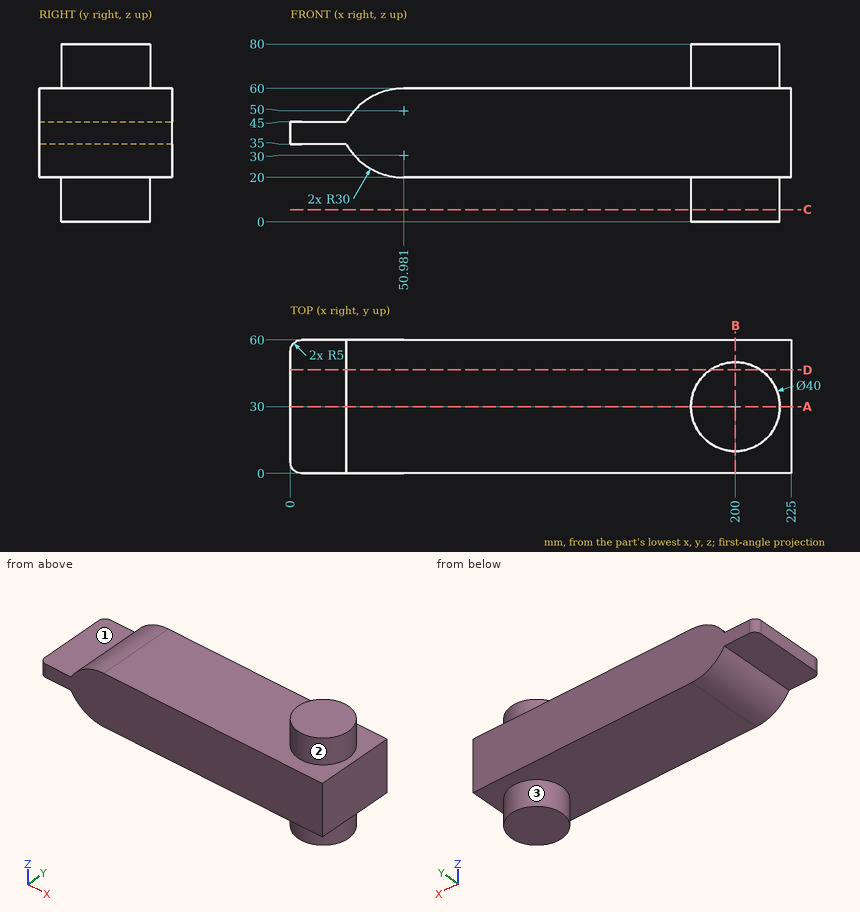
Source: three-view drawing plus pictorial views. Frame: mm from the lowest corner of the part. A direction names the side the tool comes from. Round coordinates to 2 decimals unless told otherwise and drop trailing zeros. Order: outer loops, then holes, each group sorted by start corner. A loop starts at its lowest first (then second) coordinate and runs counter-clockwise, first axis right, second up. Notation, with made-up numbers: (-38.75, -33) - (-21.75, -33) arc R20 ccw to (-21.75, -2) - close; hole circle Ø9 at (78.5, -7). An arc over 180 degrees is marked (long way). Use a Markdown table: item, result.
1. Section A-A on y = 30. Return the cut outline in (x, z).
Evaluation:
| item | result |
|---|---|
| outline | (0, 35) - (25, 35) arc R30 ccw to (50.98, 20) - (180, 20) - (180, 0) - (220, 0) - (220, 20) - (225, 20) - (225, 60) - (220, 60) - (220, 80) - (180, 80) - (180, 60) - (50.98, 60) arc R30 ccw to (25, 45) - (0, 45) - close |
2. Section C-C on z = 5.5. Return the cut outline in (x, y), then the cut area to 3 significant figures.
Evaluation:
| item | result |
|---|---|
| outline | circle Ø40 at (200, 30) |
| area | 1,260 mm^2 |
3. Section B-B on x = 200. Return the cut outline in (y, z).
Evaluation:
| item | result |
|---|---|
| outline | (0, 20) - (10, 20) - (10, 0) - (50, 0) - (50, 20) - (60, 20) - (60, 60) - (50, 60) - (50, 80) - (10, 80) - (10, 60) - (0, 60) - close |
4. Material intervals for probe 1 along Z at (x, y) = (18, 20.5); probe 2 along Z at (x, y) = (170.5, 6); probe 3 along X at (y, z) = (15.5, 8) (1 decimal), sorted ascending.
Evaluation:
| item | result |
|---|---|
| probe 1 | 35 to 45 |
| probe 2 | 20 to 60 |
| probe 3 | 186.2 to 213.8 |
5. Section D-D on y = 46.5. Return the cut outline in (x, z), then the cut area to 3 significant figures.
Evaluation:
| item | result |
|---|---|
| outline | (0, 35) - (25, 35) arc R30 ccw to (50.98, 20) - (188.7, 20) - (188.7, 0) - (211.3, 0) - (211.3, 20) - (225, 20) - (225, 60) - (211.3, 60) - (211.3, 80) - (188.7, 80) - (188.7, 60) - (50.98, 60) arc R30 ccw to (25, 45) - (0, 45) - close |
| area | 8,930 mm^2 |
6. Access query for the marked faces 1, 2 and 3. Directions: +Z, -Z, +X, -X, +Y, -Y. A direction counts if a zero-diameter tool reaches every point of the face in a straight line with its end or side. Return the directions, or none.
Evaluation:
| item | result |
|---|---|
| face 1 | +Z, -X, +Y, -Y |
| face 2 | +Z |
| face 3 | -Z |
7. First-contact query: pin 1 (7.5 mm diameter, centred on x = 17, y = 21, fed in from +Z); pin 2 (6 mm diameter, centred on x = 70, y = 13, fed in from -Z); pin 3 (3 mm diameter, centred on y = 26.5, z = 51, fed in from -X). Flat tips, straight axial feed; report the tip coordinate or a pass-through.
Evaluation:
| item | result |
|---|---|
| pin 1 | z = 45 |
| pin 2 | z = 20 |
| pin 3 | x = 28.18 |
